```python
from build123d import *

# Parameters (mm, degrees)
F0_R     = 34.925
F1_DEPTH = 19.05
F2_R     = 22.86
F3_DEPTH = 12.7
F4_R     = 34.925
F5_DEPTH = 6.35
F7_DEPTH = 6.35


with BuildPart() as f1:
    # F0 (on Front) → F1 (new body)
    with BuildSketch(Plane.XZ):
        Circle(F0_R)
    extrude(amount=-F1_DEPTH)

    # F2 (on Front) → F3 (cut)
    with BuildSketch(Plane.XZ):
        Circle(F2_R)
    extrude(amount=-F3_DEPTH, mode=Mode.SUBTRACT)

    # F4 (on Front) → F5 (join)
    with BuildSketch(Plane.XZ):
        Circle(F4_R)
    extrude(amount=F5_DEPTH)

    # F6 (on Front) → F7 (cut)
    with BuildSketch(Plane.XZ):
        with BuildLine():
            Line((12.0482778852, -8.255), (17.78, -8.255))
            Line((17.78, -8.255), (17.78, 8.255))
            Line((17.78, 8.255), (12.0482778852, 8.255))
            ThreePointArc((12.0482778852, 8.255), (13.9511849589, 4.3209331449), (14.605, 0))
            ThreePointArc((14.605, 0), (13.9511849589, -4.3209331449), (12.0482778852, -8.255))
        make_face()
        with BuildLine():
            ThreePointArc((-12.0482778852, -8.255), (0, -14.605), (12.0482778852, -8.255))
            Line((12.0482778852, -8.255), (-12.0482778852, -8.255))
        make_face()
        with BuildLine():
            Line((-12.0482778852, -8.255), (12.0482778852, -8.255))
            ThreePointArc((12.0482778852, -8.255), (13.9511849589, -4.3209331449), (14.605, 0))
            ThreePointArc((14.605, 0), (13.9511849589, 4.3209331449), (12.0482778852, 8.255))
            Line((12.0482778852, 8.255), (-12.0482778852, 8.255))
            ThreePointArc((-12.0482778852, 8.255), (-14.605, 0), (-12.0482778852, -8.255))
        make_face()
        with BuildLine():
            Line((-17.78, -8.255), (-12.0482778852, -8.255))
            ThreePointArc((-12.0482778852, -8.255), (-14.605, 0), (-12.0482778852, 8.255))
            Line((-12.0482778852, 8.255), (-17.78, 8.255))
            Line((-17.78, 8.255), (-17.78, -8.255))
        make_face()
        with BuildLine():
            Line((-12.0482778852, 8.255), (12.0482778852, 8.255))
            ThreePointArc((12.0482778852, 8.255), (0, 14.605), (-12.0482778852, 8.255))
        make_face()
    extrude(amount=F7_DEPTH, mode=Mode.SUBTRACT)


solid = f1.part
```
Geometry check sheet. Reference: the model listing, model coordinates, mm. A direction names the side the tool comes from. Coordinates: 2 decimals unless noted, no trailing zeros. Order: outer loops, then holes, each group sorted by start corner. A loop starts at its lowest first (then second) coordinate and runs counter-clockwise, first axis right, second up. Notation, with made-up numbers: M 21,46 L 48,46 A20 ccw 48,81 Z; hole C -23,24 d5. An arc over 180 degrees is marked long. One line per question, with ' | ' between items. Start each with the question number.
Item 1: Cross-section at D-D on z = 21.5. Enter the section's corners in (x, y).
Item 2: Material ranges on L1, parallel to Y at x = -7, z = 19; L2, parallel to Z at x = 0, y = 6.25 (3 decimals); L3, parallel to Y at x = 5.5, z = 7.5, recorded low to high. Write a range as [from, to].
Item 3: Cross-section at A-A on y = -2.75. Enter the section's corners in (x, z) (3 decimals), then the cut area to 3 significant figures.
Item 4: Draft check along Z on faces 4 (the flat face through (0, 0, -15)), 5 (the flat face through (0, 19.05, 0)). Enter one of: pulls with the +Z half, pulls with the -Z half, needs draft (parallel to the pull), parting line crosses it, or undercut.
Item 5: Set-up check for faces 1 (the flat face through (0, -6.35, -15)), 2 (the flat face through (-15, -3, 8.255)), 3 (the cylindrical face through (21.804, 6.261, 6.867)): record each of +Z, -Z, +X, -X, +Y, -Y from which the full face is reachable in a straight line by a thin tool's end or side.
Item 6: Cross-section at C-C on x = 0. Enter the section's corners in (y, z) (3 decimals), then the cut area to 3 significant figures.
Item 7: Gauge pin test, flat ends, axial feed: pin 1 (4.5 mm diameter, centred on x = -16, y = -3, fed in from +Z); pin 2 (6.5 mm diameter, centred on x = 15.5, y = -5, fed in from +Z); pin 3 (6 mm diameter, centred on y = 1.5, z = -14, fed in from -X). Record the tip position at first contact, or that the pin passes through.
Item 8: Cross-section at B-B on z = 0. Enter the section's corners in (x, y) (3 decimals), then the cut area to 3 significant figures.
Findings:
1) outline: M -27.52,-6.35 L 27.52,-6.35 L 27.52,19.05 L -27.52,19.05 Z; hole M -7.77,0 L 7.77,0 L 7.77,12.7 L -7.77,12.7 Z
2) L1: y = [-6.35, 0], [12.7, 19.05] | L2: z = [-34.925, -22.86], [22.86, 34.925] | L3: y = [12.7, 19.05]
3) outline: C 0,0 d69.85; hole M -17.78,-8.255 L -12.048,-8.255 A14.605 ccw 12.048,-8.255 L 17.78,-8.255 L 17.78,8.255 L 12.048,8.255 A14.605 ccw -12.048,8.255 L -17.78,8.255 Z | area: 3,030 mm²
4) face 4: undercut | face 5: needs draft
5) face 1: +Z, -Z, +X, -X, -Y | face 2: -Y | face 3: none
6) outline: M -6.35,-34.925 L 19.05,-34.925 L 19.05,34.925 L -6.35,34.925 L -6.35,14.605 L 0,14.605 L 0,22.86 L 12.7,22.86 L 12.7,-22.86 L 0,-22.86 L 0,-14.605 L -6.35,-14.605 Z | area: 1,010 mm²
7) pin 1: stops at z = 32.1 | pin 2: stops at z = 32.71 | pin 3: stops at x = -33.15
8) outline: M -34.925,-6.35 L -17.78,-6.35 L -17.78,0 L -22.86,0 L -22.86,12.7 L 22.86,12.7 L 22.86,0 L 17.78,0 L 17.78,-6.35 L 34.925,-6.35 L 34.925,19.05 L -34.925,19.05 Z | area: 968 mm²
